Here's how the part is built. I have some questions about the finished solid (model axes, mm). A direction names the side the tool comes from. Give positions to 0.01 mm unless a question says otherwise; leave off trailing zeros.
Q1. Thinking about a two-plate mould opening in X: for faces 1 (the face through (-14.721, 0.861, 16.473)), 2 (the face through (-14.67, 14.06, 1.6)), which applies, pulls with the +X half, pulls with the -X half, needs draft (parallel to the pull), parting line crosses it, or undercut?
Q2. For faces 3 (the face through (-14.661, 0.21, -0.027)), 4 (the face through (-14.72, 2.33, 15.23)), which set-ups out of +Z, -Z, +X, -X, +Y, -Y let a thin tool reach every point of the face, with its end or its side?
Q3. I'm going to push a flat-ended pin straight in: P1, Ø12, axis at x = 813.5, z = -71, coming from the +Y side. Where does the tip first touch, or does it pass through?
Q4. I need wall thicknesses on probe 1 along Z at (x, y) = (-408, 4); probe 2 along Z at (x, y) = (573, 0); probe 3 along Z at (x, y) = (-163, -12). Which ranges of each line are inside material? Lowest first, please.
```python
from build123d import *

# Parameters (mm, degrees)
F1_ANGLE_BACK = 15
F1_ANGLE      = 30


with BuildPart() as f1:
    # F0 (on Right) → F1 (revolve)
    with BuildSketch(Plane.YZ, mode=Mode.PRIVATE) as f1_sk:
        Polygon((0, 25.9807621135), (-15, 0), (15, 0), align=None)
        Polygon((0, 2.4102540378), (-10, 2.4102540378), (-3.5498759498, 13.5821966078), (-3.0693293034, 14.4145278149), (-2.5793681916, 15.2631653543), (-2.0490381057, 16.1817240079), (0, 19.7307621135), (2.0490381057, 16.1817240079), (2.5793681916, 15.2631653543), (3.0693293034, 14.4145278149), (3.5498759498, 13.5821966078), (10, 2.4102540378), align=None, mode=Mode.SUBTRACT)
        Polygon((0, 19.7307621135), (0, 16.7307621135), (1.0245190528, 16.4562430607), (2.0490381057, 16.1817240079), align=None)
        Polygon((-1.0245190528, 16.4562430607), (0, 16.7307621135), (0, 19.7307621135), (-2.0490381057, 16.1817240079), align=None)
        Polygon((2.0490381057, 16.1817240079), (1.0245190528, 16.4562430607), (1.8019436222, 15.8597042075), (2.5793681916, 15.2631653543), align=None)
        Polygon((2.4356364628, 15.1371160112), (3.0693293034, 14.4145278149), (2.5793681916, 15.2631653543), (1.8019436222, 15.8597042075), align=None)
        Polygon((2.4356364628, 15.1371160112), (3.5498759498, 13.5821966078), (3.0693293034, 14.4145278149), align=None)
        Polygon((-2.5793681916, 15.2631653543), (-3.0693293034, 14.4145278149), (-2.4356364628, 15.1371160112), (-1.8019436222, 15.8597042075), align=None)
        Polygon((-3.0693293034, 14.4145278149), (-3.5498759498, 13.5821966078), (-2.4356364628, 15.1371160112), align=None)
        Polygon((-1.8019436222, 15.8597042075), (-1.0245190528, 16.4562430607), (-2.0490381057, 16.1817240079), (-2.5793681916, 15.2631653543), align=None)
    revolve(f1_sk.sketch.rotate(Axis((0, -0.8083833382, -4000), (0, 1, 0)), -F1_ANGLE_BACK), axis=Axis((0, -0.8083833382, -4000), (0, 1, 0)), revolution_arc=F1_ANGLE)


solid = f1.part
```
Solutions:
1. face 1: undercut
1. face 2: parting line crosses it
2. face 3: -Z, +Y, -Y
2. face 4: none
3. P1: stops at y = 11.34
4. probe 1: z = -20.86 to -18.44, -7.99 to -1.71
4. probe 2: z = -41.25 to -38.82, -24.35 to -15
4. probe 3: z = -3.32 to 1.88
